```python
from build123d import *

# Parameters (mm, degrees)
F0_W      = 10.161292
F0_H      = 15.604837
F1_DEPTH  = 26.9
F2_W      = 9.254035
F2_H      = 16.512098
F3_DEPTH  = 19.9
F4_W      = 8.165322
F4_H      = 14.153226
F5_DEPTH  = 16.2
F6_R      = 23.407961
F7_DEPTH  = 22.8
F8_W      = 20.322582
F8_H      = 10.342741
F9_DEPTH  = 39.3
F11_DEPTH = 53.7
F13_DEPTH = 34.4


with BuildPart() as f1:
    # F0 (on Front) → F1 (new body)
    with BuildSketch(Plane.XZ):
        with Locations((-37.379036, -23.58871)):
            Rectangle(F0_W, F0_H)
    extrude(amount=F1_DEPTH)

    # F2 (on Front) → F3 (join)
    with BuildSketch(Plane.XZ):
        with Locations((-37.469761, -8.256049)):
            Rectangle(F2_W, F2_H)
    extrude(amount=F3_DEPTH)

    # F4 (on Front) → F5 (join)
    with BuildSketch(Plane.XZ):
        with Locations((-37.651211, 7.076613)):
            Rectangle(F4_W, F4_H)
    extrude(amount=F5_DEPTH)

    # F6 (on Front) → F7 (join)
    with BuildSketch(Plane.XZ):
        with Locations((-37.923388, -8.709677)):
            Circle(F6_R)
    extrude(amount=-F7_DEPTH)

    # F8 (on Front) → F9 (join)
    with BuildSketch(Plane.XZ):
        with Locations((-37.923389, 19.6875)):
            Rectangle(F8_W, F8_H)
    extrude(amount=-F9_DEPTH)

    # F10 (on Front) → F11 (join)
    with BuildSketch(Plane.XZ):
        Polygon((-61.027735, 27.658321), (-47.339678, 23.627182), (-28.46946, 23.277419), (-16.580516, 26.587443), (-38.470574, 36.135394), align=None)
    extrude(amount=-F11_DEPTH)

    # F12 (on Front) → F13 (join)
    with BuildSketch(Plane.XZ):
        Polygon((-18.145161, -21.592744), (-28.850807, 15.241936), (-47.721777, 15.423387), (-57.157259, -21.592744), align=None)
    extrude(amount=-F13_DEPTH)


solid = f1.part
```
CAD build for the part. Positions are in the model's coordinates, mm. A direction names the side the tool comes from. Coordinates: 2 decimals unless noted, no trailing zeros. Order: outer loops, then holes, each group sorted by start corner. A loop starts at its lowest first (then second) coordinate and runs counter-clockwise, first axis right, second up. Notation, with made-up numbers: M 82.25,5 L 117.25,5 A13 cw 117.25,30 Z; hole C -8,89 d7. An arc over 180 degrees is marked long. Answer as CSV lines item,"result".
1) Cut at D-D (x = -46). List the corners of the cut face in (y, z).
Verdict:
outline,"M 0,-30.68 L 22.8,-30.68 L 22.8,-21.59 L 34.4,-21.59 L 34.4,14.52 L 39.3,14.52 L 39.3,23.6 L 53.7,23.6 L 53.7,33.31 L 0,33.31 Z"
2) Cut at A-A (x = -56). List the corners of the cut face in (y, z), then the cut area to 3 significant figures.
Verdict:
outline,"M 0,-23.58 L 22.8,-23.58 L 22.8,-21.59 L 34.4,-21.59 L 34.4,-17.05 L 22.8,-17.05 L 22.8,6.16 L 0,6.16 Z; M 0,26.18 L 53.7,26.18 L 53.7,29.55 L 0,29.55 Z"
area,"912 mm2"
3) Flat gauge pins, fed straight in: P1, Ø4.5, axis at y = 13.5, z = 17.5, coming from the -X side; P2, Ø4, axis at x = -34.5, y = 16, coming from the +Z side; P3, Ø12.5, axis at y = -12.5, z = -24.5, coming from the -X side. Where does each tip first touch, or does it go through?
Verdict:
P1,"x = -48.08"
P2,"z = 35.28"
P3,"x = -42.46"
4) Cut at C-C (z = -2.5). List the corners of the cut face in (x, y).
Verdict:
outline,"M -60.49,0 L -42.1,0 L -42.1,-19.9 L -32.84,-19.9 L -32.84,0 L -15.35,0 L -15.35,22.8 L -23.69,22.8 L -23.69,34.4 L -52.29,34.4 L -52.29,22.8 L -60.49,22.8 Z"
5) 3-axis set-ups, long thin cutter, end or side, ignore diameter. For faces 1 (the flat face through (-38, -16.2, 7)), 2 (the flat face through (-27.762, 19, 19)), 3 (the flat face through (-42.097, -10, -8)), 4 (the flat face through (-20, 22.8, -4)): which of +Z, -Z, +X, -X, +Y, -Y reach the whole face in a straight line?
Verdict:
face 1,"+Z, +X, -X, -Y"
face 2,"+X, +Y, -Y"
face 3,"+Z, -X, -Y"
face 4,"+X, +Y"
6) Drill centre lines: L1, parallel to Y at x = -27, z = -0.5; L2, parallel to Z at x = -40, y = -21; L3, parallel to X at y = 20, z = -9.5. Where is each one in solid material? Low to high. Write a range as from..to.
Verdict:
L1,"0..34.4"
L2,"-31.39..-15.79"
L3,"-61.32..-14.53"
7) Cut at B-B (y = 30.5). List the corners of the cut face in (x, z).
Verdict:
outline,"M -61.03,27.66 L -48.08,23.85 L -48.08,14.52 L -47.95,14.52 L -57.16,-21.59 L -18.15,-21.59 L -28.64,14.52 L -27.76,14.52 L -27.76,23.47 L -16.58,26.59 L -38.47,36.14 Z"
8) Mould opens along Z. For faces 5 (the flat face through (-37, -26.9, -23)), 6 (the flat face through (-27.372, 26.474, 31.295)), 7 (the flat face through (-23.757, 27.312, -2.285)) say: released by +Z, released by -Z, zero draft, split by the parting line, or undercut.
Verdict:
face 5,"zero draft"
face 6,"released by +Z"
face 7,"undercut"
